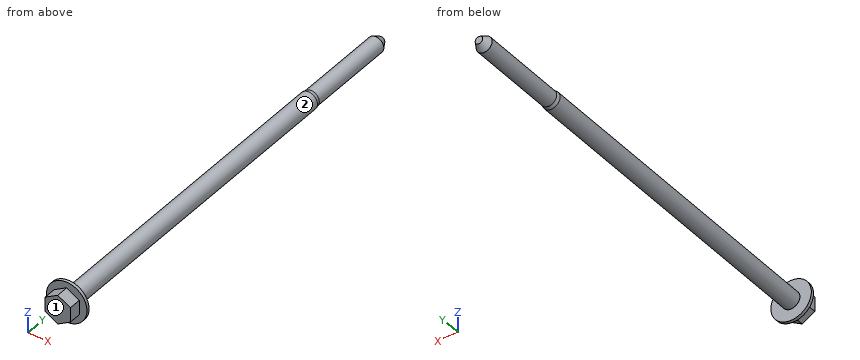
from build123d import *

# Parameters (mm, degrees)
BOSS_EXTRUDE1_DEPTH = 3.4
SKETCH2_R           = 5.48
BOSS_EXTRUDE2_DEPTH = 0.83
SKETCH3_R           = 2.385
BOSS_EXTRUDE3_DEPTH = 92
SKETCH4_R           = 2.165
BOSS_EXTRUDE4_DEPTH = 26.5
CHAMFER1_SIZE       = 2
CHAMFER1_SIZE2      = 1.154700538
CHAMFER2_SIZE       = 1
CHAMFER2_SIZE2      = 0.212556562


with BuildPart() as part:
    # Sketch1 → Boss-Extrude1 (new body)
    with BuildSketch(Plane(origin=(0, 0, 0), x_dir=(1, 0, 0), z_dir=(0, 1, 0))):
        Polygon((0, -3.937528836), (3.41, -1.968764418), (3.41, 1.968764418), (0, 3.937528836), (-3.41, 1.968764418), (-3.41, -1.968764418), align=None)
    extrude(amount=BOSS_EXTRUDE1_DEPTH)

    # Sketch2 → Boss-Extrude2 (add)
    with BuildSketch(Plane(origin=(0, 3.4, 0), x_dir=(1, 0, 0), z_dir=(0, 1, 0))):
        Circle(SKETCH2_R)
    extrude(amount=BOSS_EXTRUDE2_DEPTH)

    # Sketch3 → Boss-Extrude3 (add)
    with BuildSketch(Plane(origin=(0, 4.23, 0), x_dir=(1, 0, 0), z_dir=(0, 1, 0))):
        Circle(SKETCH3_R)
    extrude(amount=BOSS_EXTRUDE3_DEPTH)

    # Sketch4 → Boss-Extrude4 (add)
    with BuildSketch(Plane(origin=(0, 96.23, 0), x_dir=(1, 0, 0), z_dir=(0, 1, 0))):
        Circle(SKETCH4_R)
    extrude(amount=BOSS_EXTRUDE4_DEPTH)

    # Chamfer1
    chamfer1_edges = [part.edges().sort_by_distance(p)[0] for p in [
        (-2.165, 122.73, 0),
    ]]
    chamfer1_side = [part.faces().sort_by_distance(p)[0] for p in [
        (-2.165, 109.48, 0),
    ]]
    chamfer(chamfer1_edges, length=CHAMFER1_SIZE, length2=CHAMFER1_SIZE2, reference=chamfer1_side[0])

    # Chamfer2
    chamfer2_edges = [part.edges().sort_by_distance(p)[0] for p in [
        (-2.385, 96.23, 0),
    ]]
    chamfer2_side = [part.faces().sort_by_distance(p)[0] for p in [
        (-2.385, 50.23, 0),
    ]]
    chamfer(chamfer2_edges, length=CHAMFER2_SIZE, length2=CHAMFER2_SIZE2, reference=chamfer2_side[0])


solid = part.part
Work out the finished part from the listing and answer in its coordinate system (mm). Face numbers are marked on the shaded views. A direction names the side the tool comes from. Coordinates: 2 decimals unless noted, no trailing zeros. Loops run counter-clockwise (first coordinate to the right, second up) from the corner with the lowest first, then second, coordinate; pieces in that order, holes last. Notation, with made-up numbers: M 15.5,54 L 64.5,54 A31 ccw 64.5,87 Z; hole C 22.25,58 d9. An arc over 180 degrees is marked long. Answer in a Markdown table with one row per item. Add a question column.
1. Find section C-C, the plane y = 18. Write down the section's boundary in (x, z) (3 decimals), then the cut area to 3 significant figures.
2. Flat-ended cylindrical pins translate along their axes: P1, Ø3, axis at x = -0.5, y = 37, coming from the -Z side (3 decimals); P2, Ø1.5, axis at x = -2, y = 44.5, coming from the +Z side; P3, Ø5, axis at y = 83, z = 4, coming from the -X side. Find the tip coordinate at first contact, or state that the pin passes through.
3. Consider L1, parallel to Z at x = -1, y = 41.5; L2, parallel to Y at x = 2.25, z = 2.75. Determine where each line is inside the solid, lowest interval first.
4. Find section A-A, the plane z = 0. Write down the section's boundary in (x, y) (3 decimals), then the cut area to 3 significant figures.
5. A tool of negligible diameter and unlimited length cuts with its end or side. For the marked faces 1 and 2, from which of +Z, -Z, +X, -X, +Y, -Y can it reach the whole face along a straight path? Write none if from no direction.
6. Find section B-B, the plane y = 115.5. Write down the section's boundary in (x, z) (3 decimals), then the cut area to 3 significant figures.
Reported:
| question | item | result |
|---|---|---|
| 1 | outline | C 0,0 d4.77 |
| 1 | area | 17.9 mm^2 |
| 2 | P1 | stops at z = -2.385 |
| 2 | P2 | stops at z = 2.03 |
| 2 | P3 | stops at x = -1.85 |
| 3 | L1 | z = -2.17 to 2.17 |
| 3 | L2 | y = 3.4 to 4.23 |
| 4 | outline | M -5.48,3.4 L -3.41,3.4 L -3.41,0 L 3.41,0 L 3.41,3.4 L 5.48,3.4 L 5.48,4.23 L 2.385,4.23 L 2.385,95.23 L 2.172,96.23 L 2.165,96.23 L 2.165,120.73 L 1.01,122.73 L -1.01,122.73 L -2.165,120.73 L -2.165,96.23 L -2.172,96.23 L -2.385,95.23 L -2.385,4.23 L -5.48,4.23 Z |
| 4 | area | 583 mm^2 |
| 5 | face 1 | +Z, -Z, +X, -X, -Y |
| 5 | face 2 | +Y |
| 6 | outline | C 0,0 d4.33 |
| 6 | area | 14.7 mm^2 |
